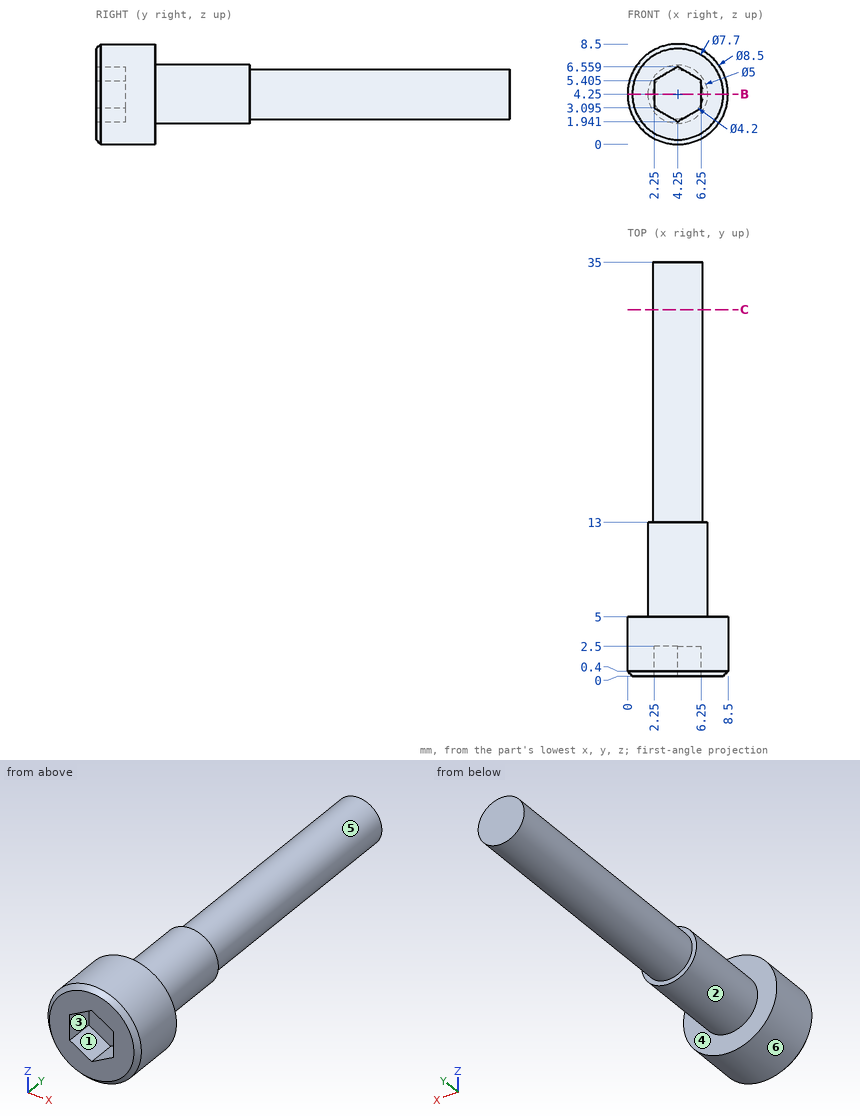
Here's the drawing with two shaded views (mm, measured from the low corner). I have some questions. A direction names the side the tool comes from. Give positions to 0.01 mm unless a question says otherwise; leave off trailing zeros. Order: outer loops, then holes, each group sorted by start corner. A loop starts at its lowest first (then second) coordinate and runs counter-clockwise, first axis right, second up. Notation, with made-up numbers: (-6.75, 0.5) -> (28.25, 0.5) arc R19 cw to (28.25, 25.5) -> close; hole circle Ø5 at (48, -6.75). An arc over 180 degrees is marked (long way). Use a Markdown table: item, result. Add a question column.
Item 1: Will these pins go through, and if not, where does the flat tip stop? pin 1 (2 mm diameter, centred on x = 4, z = 4, fed in from -Y); pin 2 (3 mm diameter, centred on x = 4.5, y = 30, fed in from -Z); pin 3 (1 mm diameter, centred on x = 5.5, y = 11, fed in from +Z) (1 decimal); pin 4 (1.2 mm diameter, centred on y = 1.5, z = 4, fed in from -X).
Item 2: Imagine slicing it at B-B on z = 4.25. Please give me the cut outline in (x, y).
Item 3: I need wall thicknesses on line 1 (Y direction, x = 1.75, z = 2.75); line 2 (X direction, y = 10, z = 2.75); line 3 (Y direction, x = 4, z = 5.5). Which ranges of each line are inside material? Lowest first, please.
Item 4: If we mould it in two halves opening along X, with no side actions, what happens to the marked faces 1, 2, 3 and 4? For each: pulls with the +X half, pulls with the -X half, needs draft (parallel to the pull), parting line crosses it, or undercut.
Item 5: Imagine slicing it at C-C on y = 31. Please give me the cut outline in (x, z).
Item 6: For the marked faces 5 and 6, which set-ups out of +Z, -Z, +X, -X, +Y, -Y let a thin tool reach every point of the face, with its end or its side?
Data:
| question | item | result |
|---|---|---|
| 1 | pin 1 | stops at y = 2.5 |
| 1 | pin 2 | stops at z = 2.15 |
| 1 | pin 3 | stops at z = 6.6 |
| 1 | pin 4 | stops at x = 0 |
| 2 | outline | (0, 0.4) -> (0.4, 0) -> (2.25, 0) -> (2.25, 2.5) -> (6.25, 2.5) -> (6.25, 0) -> (8.1, 0) -> (8.5, 0.4) -> (8.5, 5) -> (6.75, 5) -> (6.75, 13) -> (6.35, 13) -> (6.35, 35) -> (2.15, 35) -> (2.15, 13) -> (1.75, 13) -> (1.75, 5) -> (0, 5) -> close |
| 3 | line 1 | y = 0 to 5 |
| 3 | line 2 | x = 2.25 to 6.25 |
| 3 | line 3 | y = 2.5 to 35 |
| 4 | face 1 | undercut |
| 4 | face 2 | parting line crosses it |
| 4 | face 3 | undercut |
| 4 | face 4 | needs draft |
| 5 | outline | circle Ø4.2 at (4.25, 4.25) |
| 6 | face 5 | +Y |
| 6 | face 6 | +Y, -Y |
